```python
from build123d import *

# Parameters (mm, degrees)
SKETCH3_R                = 27.5
SKETCH3_R_2              = 25
CUT_EXTRUDE1_DEPTH       = 2
SKETCH4_W                = 78
SKETCH4_H                = 82
SKETCH4_W_2              = 42
SKETCH4_H_2              = 42
BOSS_EXTRUDE1_DEPTH      = 5
M4_CLEARANCE_HOLE1_D     = 4.5
M4_CLEARANCE_HOLE1_DEPTH = 5
BOSS_EXTRUDE4_DEPTH      = 5
FILLET1_R                = 25


with BuildPart() as part:
    # Sketch2 → Revolve1 (revolve)
    with BuildSketch(Plane.XY):
        Polygon((0, 21), (35, 21), (35, 15), (39, 15), (39, 16), (55, 16), (55, 26), (28, 26), (28, 28), (0, 28), align=None)
    revolve(axis=Axis((-64.103352454, 0, 0), (1, 0, 0)))

    # Sketch3 → Cut-Extrude1 (cut)
    with BuildSketch(Plane(origin=(53, 0, 0), x_dir=(0, 0, -1), z_dir=(1, 0, 0))):
        Circle(SKETCH3_R)
        Circle(SKETCH3_R_2, mode=Mode.SUBTRACT)
    extrude(amount=CUT_EXTRUDE1_DEPTH, mode=Mode.SUBTRACT)

    # Sketch4 → Boss-Extrude1 (add)
    with BuildSketch(Plane.ZY):
        Rectangle(SKETCH4_W, SKETCH4_H)
        Rectangle(SKETCH4_W_2, SKETCH4_H_2, mode=Mode.SUBTRACT)
    extrude(amount=BOSS_EXTRUDE1_DEPTH)

    # M4 Clearance Hole1
    with Locations(Plane.ZY.offset(5)):
        with Locations((-27, 25), (27, 25), (27, -29), (-27, -29)):
            Hole(M4_CLEARANCE_HOLE1_D / 2, depth=M4_CLEARANCE_HOLE1_DEPTH)

    # Sketch11 → Boss-Extrude4 (add)
    with BuildSketch(Plane.ZY):
        Polygon((-21, 18), (-18, 21), (-21, 21), align=None)
        Polygon((21, 21), (21, 18), (18, 21), align=None)
        Polygon((21, -21), (21, -18), (18, -21), align=None)
        Polygon((-21, -21), (-21, -18), (-18, -21), align=None)
    extrude(amount=BOSS_EXTRUDE4_DEPTH)

    # Fillet1
    fillet1_edges = [part.edges().sort_by_distance(p)[0] for p in [
        (-2.5, 41, -39),
        (-2.5, -41, -39),
    ]]
    fillet(fillet1_edges, radius=FILLET1_R)


solid = part.part
```
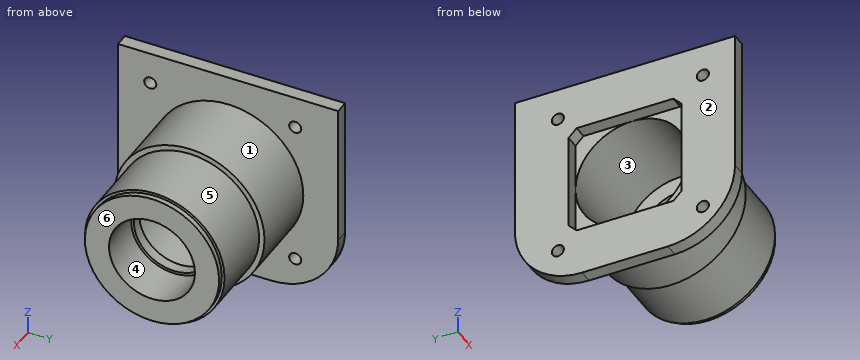
Part model, mm, in its own coordinate system. Face numbers are marked on the shaded views. A direction names the side the tool comes from. Give positions to 0.01 mm unless a question says otherwise; leave off trailing zeros. Order: outer loops, then holes, each group sorted by start corner. A loop starts at its lowest first (then second) coordinate and runs counter-clockwise, first axis right, second up. Notation, with made-up numbers: (36, -24) - (71, -24) arc R35 cw to (71, 8) - close; hole circle Ø1 at (75.5, 88). An arc over 180 degrees is marked (long way). Use one line per item in the form item = value.
Item 1: Probe probe 1 along Y at (x, z) = (-1, 27); probe 2 along Z at (x, y) = (37, 0); probe 3 along Z at (x, y) = (17, 0). List the from-to ranges inside material, lowest first. Write a range as from..to.
Solution:
probe_1 = -41..-31.25, -26.75..22.75, 27.25..41
probe_2 = -26..-15, 15..26
probe_3 = -28..-21, 21..28
Item 2: Slice it at D-D on y = -36. Give the cut face in (x, z).
Solution:
outline = (-5, -29) - (0, -29) - (0, 39) - (-5, 39) - close
Item 3: Which spindle directions (+Z, -Z, +X, -X, +Y, -Y) get a long thin tool onto all of the face, cutting with end or side? Do the marked faces 1, 2 and 3. Say none if no direction does.
Solution:
face_1 = +X
face_2 = +Z, -Z, -X, +Y, -Y
face_3 = -X
Item 4: Slice it at C-C on x = 17.5. Give the cut face in (y, z).
Solution:
outline = circle Ø56 at (0, 0); hole circle Ø42 at (0, 0)
Item 5: Pin check, flat tips, straight feed: pin 1 Ø2.5 at (y, z) = (25, 27) entering from +X; pin 2 Ø2 at (y, z) = (12, 12) entering from -X; pin 3 Ø6 at (y, z) = (-29, 27) entering from +X; pin 4 Ø23 at (y, z) = (-14.5, 6) entering from -X. Stop position of each tip, or through.
Solution:
pin_1 = through
pin_2 = 35
pin_3 = 0
pin_4 = -5
Item 6: Two-plate mould, pull along Y, no slides. Class the marked faces 4, 5 and 6: released by +Y, released by -Y, zero draft, split by the parting line, or undercut.
Solution:
face_4 = undercut
face_5 = split by the parting line
face_6 = zero draft
